```python
from build123d import *

# Parameters (mm, degrees)
F0_W     = 127
F0_H     = 76.2
F1_DEPTH = 203.2
F2_R     = 5.08
F3_R     = 0.635
F4_DEPTH = 50.8
F5_W     = 50.8
F5_H     = 76.2
F5_R     = 12.7
F6_DEPTH = 5.08


with BuildPart() as f1:
    # F0 (on Front) → F1 (new body)
    with BuildSketch(Plane.XZ):
        with Locations((63.5, 38.1)):
            Rectangle(F0_W, F0_H)
    extrude(amount=F1_DEPTH)

    # F2
    f2_edges = [f1.edges().sort_by_distance(p)[0] for p in [
        (63.5, -203.2, 76.2),
        (127, -101.6, 76.2),
        (127, -203.2, 38.1),
        (127, 0, 38.1),
        (127, -101.6, 0),
        (63.5, -203.2, 0),
        (63.5, 0, 0),
        (0, 0, 38.1),
        (0, -101.6, 0),
        (0, -101.6, 76.2),
        (63.5, 0, 76.2),
    ]]
    fillet(f2_edges, radius=F2_R)

    # F3 (on face) → F4 (join)
    with BuildSketch(Plane.XZ.offset(203.2)):
        with Locations((22.490209, 13.902469)):
            Circle(F3_R)
        with Locations((35.190209, 13.902469)):
            Circle(F3_R)
        with Locations((47.890209, 13.902469)):
            Circle(F3_R)
    extrude(amount=F4_DEPTH)

    # F5 (on face) → F6 (join)
    with BuildSketch(Plane.XY.offset(76.2)):
        with Locations((55.88, -68.58)):
            Rectangle(F5_W, F5_H)
        with Locations((33.02, -147.32)):
            Circle(F5_R)
        with Locations((83.82, -147.32)):
            Circle(F5_R)
    extrude(amount=F6_DEPTH)


solid = f1.part
```
Source: CAD feature listing. Evaluate the final solid. Frame: model axes, mm. A direction names the side the tool comes from. Coordinates: 2 decimals unless noted, no trailing zeros. Loops run counter-clockwise (first coordinate to the right, second up) from the corner with the lowest first, then second, coordinate; pieces in that order, holes last. Notation, with made-up numbers: (53, 70.5) -> (69, 70.5) arc R27 cw to (69, 97.5) -> close; hole circle Ø7 at (6, 0.5). An arc over 180 degrees is marked (long way). One line per item, written item: value. Start each with the question number.
Q1. Section query B-B, the plane y = -178. Return the cut outline in (x, z), and give its area (3 significant figures).
Q2. Section query C-C, the plane z = 49. Return the cut outline in (x, y).
Q3. Mould query, pull axis Y, two halves, no side actions, for faces 3 (the face through (63, 0, 39)), 4 (the face through (56, -68, 81.28)), 5 (the face through (71.132, -146.762, 78.704)). Classes: pulls with the +Y half, pulls with the -Y half, needs draft (parallel to the pull), parting line crosses it, or undercut.
Q4. Section query A-A, the plane x = 83.82. Return the cut outline in (y, z).
Q5. Contact query for flat-ended pins moving along their axis: P1, Ø1.5, axis at x = 50.5, z = 80, coming from the +Y side; P2, Ø8, axis at x = 71, z = 32, coming from the -Y side; P3, Ø2.5, axis at x = 57, z = 78, coming from the -Y side. Output: stop coordinate, or through.
Q6. Line query: line 1 along Y through (x, z) = (30, 8); line 2 along Z through (x, y) = (18.5, -62.5); line 3 along X through (y, z) = (-128, 72.5). Output: solid intervals per line, ascending.
Q7. Set-up query: faces 1 (the face through (125.551, -1.528, 38.562)), 2 (the face through (81.28, -69, 79)). Return all of +Z, -Z, +X, -X, +Y, -Y with unobstructed straight access to the full face (end or side cutting, diameter ignored); none if empty.
Q8. Section query D-D, the plane x = 104. Return the cut outline in (y, z), and give its area (3 significant figures).
Results:
1. outline: (0, 5.08) arc R5.08 ccw to (5.08, 0) -> (121.92, 0) arc R5.08 ccw to (127, 5.08) -> (127, 71.12) arc R5.08 ccw to (121.92, 76.2) -> (5.08, 76.2) arc R5.08 ccw to (0, 71.12) -> close
1. area: 9,660 mm^2
2. outline: (0, -203.2) -> (121.92, -203.2) arc R5.08 ccw to (127, -198.12) -> (127, -5.08) arc R5.08 ccw to (121.92, 0) -> (5.08, 0) arc R5.08 ccw to (0, -5.08) -> close
3. face 3: pulls with the +Y half
3. face 4: needs draft
3. face 5: undercut
4. outline: (-203.2, 5.08) arc R5.08 ccw to (-198.12, 0) -> (-5.08, 0) arc R5.08 ccw to (0, 5.08) -> (0, 71.12) arc R5.08 ccw to (-5.08, 76.2) -> (-134.62, 76.2) -> (-134.62, 81.28) -> (-160.02, 81.28) -> (-160.02, 76.2) -> (-198.12, 76.2) arc R5.08 ccw to (-203.2, 71.12) -> close
5. P1: y = -30.48
5. P2: y = -203.2
5. P3: y = -106.68
6. line 1: -203.2 to 0
6. line 2: 0 to 76.2
6. line 3: 0.19 to 126.81
7. face 1: +Z, -Z, +X, +Y
7. face 2: +Z, +X, +Y
8. outline: (-203.2, 5.08) arc R5.08 ccw to (-198.12, 0) -> (-5.08, 0) arc R5.08 ccw to (0, 5.08) -> (0, 71.12) arc R5.08 ccw to (-5.08, 76.2) -> (-198.12, 76.2) arc R5.08 ccw to (-203.2, 71.12) -> close
8. area: 15,500 mm^2
